Design review of the part built by this model. Coordinates are the model's own, in mm. A direction names the side the tool comes from. Give positions to 0.01 mm unless a question says otherwise; leave off trailing zeros. Write each loop counter-clockwise with the first axis right and the second up, starting at its lowest first coordinate (ties: lowest second). Pieces come first, ordered by that corner, then holes. Notation, with made-up numbers: M -31,82.5 L 25,82.5 A22 cw 25,92.5 Z; hole C -15,25.25 d1. An arc over 180 degrees is marked long. Write each question's results on one line, items separated by ' | '. Start each with the question number.
from build123d import *

# Parameters (mm, degrees)
SKETCH_1_R      = 1.6
EXTRUDE_1_DEPTH = 5
EXTRUDE_2_DEPTH = 60
FILLET_2_R      = 10
FILLET_3_R      = 10


with BuildPart() as part:
    # 草图1 → 凸台-拉伸1 (new body)
    with BuildSketch(Plane(origin=(0, 0, 0), x_dir=(1, 0, 0), z_dir=(0, 1, 0))):
        with BuildLine():
            ThreePointArc((-10.870399894, 40.568884704), (0, 42), (10.870399894, 40.568884704))
            Line((10.870399894, 40.568884704), (19.411428383, 72.444436972))
            Line((19.411428383, 72.444436972), (0, 90))
            Line((0, 90), (-19.411428383, 72.444436972))
            Line((-19.411428383, 72.444436972), (-10.870399894, 40.568884704))
        make_face()
        with Locations(Location((0, 65, 0), (0, 0, 270))):
            Circle(SKETCH_1_R, mode=Mode.SUBTRACT)
        with Locations(Location((0, 48.92241394, 0), (0, 0, 270))):
            Circle(SKETCH_1_R, mode=Mode.SUBTRACT)
    extrude(amount=EXTRUDE_1_DEPTH)

    # 草图5 → 凸台-拉伸2 (add)
    with BuildSketch(Plane(origin=(0, 5, 0), x_dir=(1, 0, 0), z_dir=(0, 1, 0))):
        with BuildLine():
            Line((0, 90), (-6.925726506, 74.679544136))
            ThreePointArc((-6.925726506, 74.679544136), (0, 75), (6.925726506, 74.679544136))
            Line((6.925726506, 74.679544136), (0, 90))
        make_face()
    extrude(amount=EXTRUDE_2_DEPTH)

    # 旋转1: read off the stored shape, not the designer's step
    # 旋转1: loft between two sections, ruled curve by curve
    revolve_1_from = [
        Edge.make_three_point_arc((1e-09, 34.818833313, -84.706290842), (-3.706290842, 34.818833313, -81.000000001), (0, 34.818833313, -77.293709158)),
        Edge.make_three_point_arc((0, 34.818833313, -77.293709158), (3.706290842, 34.818833313, -81), (1e-09, 34.818833313, -84.706290842)),
    ]
    revolve_1_to = [
        Edge.make_three_point_arc((3e-09, 65, -98.78), (-17.78, 65, -81.000000003), (-2e-09, 65, -63.22)),
        Edge.make_three_point_arc((-2e-09, 65, -63.22), (17.78, 65, -80.999999999), (3e-09, 65, -98.78)),
    ]
    revolve_1 = Solid(Shell([*[Face.make_surface_from_curves(revolve_1_from[k], revolve_1_to[k]) for k in range(2)], Face(Wire(revolve_1_from)), Face(Wire(revolve_1_to))]))
    add(revolve_1)

    # 圆角2
    # the kernel refuses this fillet: 10 mm, written as the material it adds along each edge
    with BuildSketch(Plane(origin=(17.223805664, 5, -51.899079574), x_dir=(0.9112185824712705, 0, -0.4119231663296544), z_dir=(-0.4119231663296544, 0, -0.9112185824712706))) as fillet_2_piece_1_section:
        with BuildLine():
            CenterArc((FILLET_2_R, -FILLET_2_R), FILLET_2_R, 90, 90)
            Line((0, -FILLET_2_R), (0, 0))
            Line((0, 0), (FILLET_2_R, 0))
        make_face()
    fillet_2_piece_1 = extrude(amount=66.813151267, mode=Mode.PRIVATE)
    fillet_2_piece_1 = split(fillet_2_piece_1, bisect_by=Plane(origin=(28.429094155, 5, -64.28892174), z_dir=(-0.6707629255291222, 0, 0.7416718261708566)), keep=Keep.TOP, mode=Mode.PRIVATE)
    fillet_2_piece_1 = split(fillet_2_piece_1, bisect_by=Plane(origin=(-11.378711034, 5, -64.829060887), z_dir=(0.9112185824712704, 0, 0.411923166329655)), keep=Keep.TOP, mode=Mode.PRIVATE)
    fillet_2_piece_1 = fillet_2_piece_1 - Plane(origin=(0, 5, 0), x_dir=(-0.09234302007576177, 0, -0.9957272551473558), z_dir=(0, -1, 0)) * Cylinder(75, 174, mode=Mode.PRIVATE)
    add(fillet_2_piece_1)

    # 圆角3
    # the kernel refuses this fillet: 10 mm, written as the material it adds along each edge
    with BuildSketch(Plane(origin=(10.298079158, 5, -112.780464562), x_dir=(-0.9112185824712703, 0, -0.41192316632965503), z_dir=(-0.411923166329655, 0, 0.9112185824712704))) as fillet_3_piece_1_section:
        with BuildLine():
            CenterArc((FILLET_3_R, -FILLET_3_R), FILLET_3_R, 90, 90)
            Line((0, -FILLET_3_R), (0, 0))
            Line((0, 0), (FILLET_3_R, 0))
        make_face()
    fillet_3_piece_1 = extrude(amount=66.813151267, mode=Mode.PRIVATE)
    fillet_3_piece_1 = split(fillet_3_piece_1, bisect_by=Plane(origin=(16.997698866, 5, -105.372602567), z_dir=(0.6707629255291219, 0, 0.7416718261708569)), keep=Keep.TOP, mode=Mode.PRIVATE)
    fillet_3_piece_1 = fillet_3_piece_1 - Plane(origin=(0, 5, 0), x_dir=(-0.0923430200760307, 0, -0.995727255147331), z_dir=(0, -1, 0)) * Cylinder(75, 174, mode=Mode.PRIVATE)
    fillet_3_piece_1 = split(fillet_3_piece_1, bisect_by=Plane(origin=(-5.668223875, 5, -95.126302894), z_dir=(-0.6707629255289835, 0, 0.7416718261709819)), keep=Keep.TOP, mode=Mode.PRIVATE)
    add(fillet_3_piece_1)


solid = part.part
Q1. For pin 1 Ø3 at (x, z) = (0, -65) entering from -Y; pin 2 Ø1.5 at (y, z) = (9.5, -75.5) entering from +X; pin 3 Ø6 at (x, y) = (7.5, 45.5) entering from -Z, all flat-tipped, find the tip position at first contact; note any pin that passes through.
Q2. For faces 4 (the cylindrical face through (6.6, 9.2, -79.9)), 5 (the cylindrical face through (0.481, 2.465, -63.474)), 6 (the cylindrical face through (0.481, 2.465, -47.396)), 7 (the cylindrical face through (-6.503, 9.175, -80.159)), list the 3-axis set-ups (+Z, -Z, +X, -X, +Y, -Y) from which the entire face can be reached by the end or side of a thin tool; tool diameter is ignored.
Q3. We need section A-A on z = -65. Count the separate pieces of the cut face and the enclosed holes in it, and give its area (3 significant figures).
Q4. Wall thickness on line 1 along Y through (x, z) = (14, -57); line 2 along X through (y, z) = (2, -65); line 3 along X through (y, z) = (42, -84): over which ranges is each line inside the solid? List them lowest first. Write a range as from..to.
Q5. We need section B-B on y = 32. Write out the cut boundary in (x, z).
Q6. The part is to be moulded in two halves that separate along X. For faces 1 (the cylindrical face through (0, 2, -42)), 2 (the flat face through (0, 0, -60)), 3 (the flat face through (15.08, 2.46, -56.28)), say which applies: pulls with the +X half, pulls with the -X half, needs draft (parallel to the pull), parting line crosses it, or undercut.
Answer sheet:
1) pin 1: y = 57.97 | pin 2: x = 9.05 | pin 3: z = -89.05
2) face 4: -Z, +X | face 5: -Y | face 6: +Y, -Y | face 7: -Z, -X
3) separate pieces: 3 | enclosed holes: 0 | area: 197 mm^2
4) line 1: 0..5 | line 2: -17.42..-1.6, 1.6..17.42 | line 3: -6.39..6.39
5) outline: M -6.93,-74.68 L 0,-90 L 6.93,-74.68 A75 cw Z
6) face 1: undercut | face 2: needs draft | face 3: pulls with the +X half
